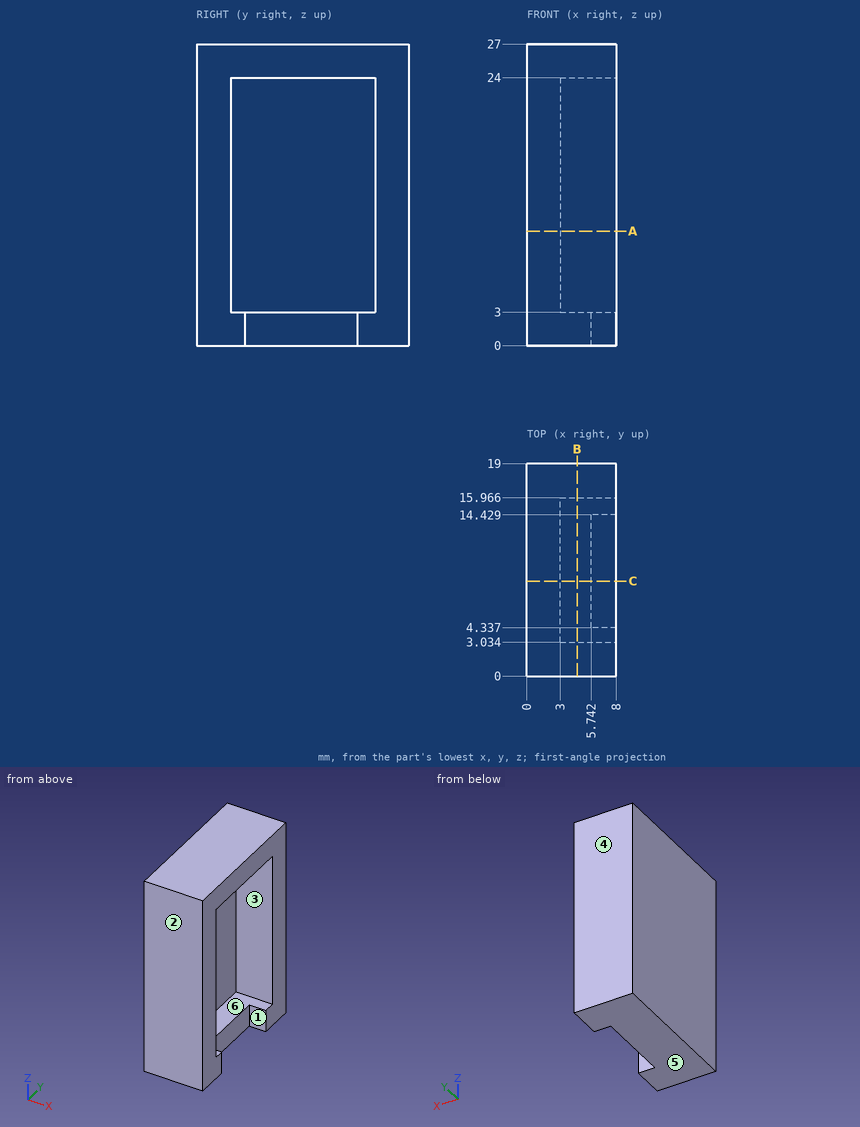
Drawing for the job (mm, zero at the part's lowest x, y, z). A direction names the side the tool comes from. Round coordinates to 2 decimals unless told otherwise and drop trailing zeros. Loops run counter-clockwise (first coordinate to the right, second up) from the corner with the lowest first, then second, coordinate; pieces in that order, holes last. Notation, with made-up numbers: M 1,29.5 L 22,29.5 A26 cw 22,61.5 Z; hole C 15,60 d5. An arc over 180 degrees is marked long. Use a Markdown table: item, result. Add a question column.
(1) Cut at A-A (z = 10.25). Give the cut face in (x, y) (1 decimal).
(2) Pull direction Y, two halves, no side cores. Call the marked faces 4, 5 and 6: +Y half, -Y half, draft (parallel to the pull), parting line (faces both ways), or undercut.
(3) Flat gauge pins, fed straight in: pin 1 (3 mm diameter, centred on x = 6.5, z = 21, fed in from -Y); pin 2 (0.9 mm diameter, centred on y = 11.5, z = 1, fed in from +X). Where does each tip first touch, or does it go through?
(4) Cut at C-C (y = 8.5). Give the cut face in (x, z).
(5) Which spindle directions (+Z, -Z, +X, -X, +Y, -Y) get a long thin tool onto all of the face, cutting with end or side? Do the marked faces 1, 2 and 3. Say none if no direction does.
(6) Drill centre lines: line 1 (Z direction, x = 4.5, y = 15); line 2 (Y direction, x = 7.5, z = 5.75) (1 decimal); line 3 (Z direction, x = 7, y = 8.25). Where is each one in solid material? Low to high.
(7) Cut at B-B (x = 4.5). Give the cut face in (y, z) (1 decimal).
Geometry says:
| question | item | result |
|---|---|---|
| 1 | outline | M 0,0 L 8,0 L 8,3 L 3,3 L 3,16 L 8,16 L 8,19 L 0,19 Z |
| 2 | face 4 | +Y half |
| 2 | face 5 | draft |
| 2 | face 6 | undercut |
| 3 | pin 1 | stops at y = 0 |
| 3 | pin 2 | stops at x = 5.74 |
| 4 | outline | M 0,0 L 5.74,0 L 5.74,3 L 3,3 L 3,24 L 8,24 L 8,27 L 0,27 Z |
| 5 | face 1 | -Z, +X |
| 5 | face 2 | +Z, -Z, +X, -X, -Y |
| 5 | face 3 | +X |
| 6 | line 1 | z = 0 to 3, 24 to 27 |
| 6 | line 2 | y = 0 to 3, 16 to 19 |
| 6 | line 3 | z = 24 to 27 |
| 7 | outline | M 0,0 L 19,0 L 19,27 L 0,27 Z; hole M 3,3 L 16,3 L 16,24 L 3,24 Z |
